from build123d import *

# Parameters (mm, degrees)
BOSS_EXTRUDE1_DEPTH      = 13
BOSS_EXTRUDE1_DEPTH_BACK = 13
SKETCH1_W                = 142.3
SKETCH1_H                = 46.5
FILLET1_R                = 1.5
SKETCH2_R                = 2.25
BOSS_EXTRUDE2_DEPTH      = 18.5
SKETCH3_R                = 0.75
BOSS_EXTRUDE3_DEPTH      = 9


with BuildPart() as part:
    # Sketch1 → Boss-Extrude1 (new, two sides: drawn at the far end of the back side and taken through both)
    with BuildSketch(Plane.XY.offset(-BOSS_EXTRUDE1_DEPTH_BACK)):
        Rectangle(SKETCH1_W, SKETCH1_H)
    extrude(amount=BOSS_EXTRUDE1_DEPTH + BOSS_EXTRUDE1_DEPTH_BACK)

    # Fillet1
    fillet1_edges = [part.edges().sort_by_distance(p)[0] for p in [
        (-71.15, 0, 13),
        (71.15, 0, -13),
        (0, -23.25, 13),
        (71.15, 0, 13),
        (0, 23.25, 13),
        (0, 23.25, -13),
        (-71.15, 0, -13),
        (-71.15, 23.25, 0),
        (71.15, 23.25, 0),
        (71.15, -23.25, 0),
        (-71.15, -23.25, 0),
        (0, -23.25, -13),
    ]]
    fillet(fillet1_edges, radius=FILLET1_R)

    # Sketch2 → Boss-Extrude2 (add)
    with BuildSketch(Plane.XY.offset(13)):
        with Locations(Location((-66.4, -18.25, 0), (0, 0, 180))):
            Circle(SKETCH2_R)
        with Locations(Location((-66.4, -13.25, 0), (0, 0, 180))):
            Circle(SKETCH2_R)
    extrude(amount=BOSS_EXTRUDE2_DEPTH)

    # Sketch3 → Boss-Extrude3 (add)
    with BuildSketch(Plane.XY.offset(13)):
        with Locations(Location((-67.9, 19.5, 0), (0, 0, 180))):
            Circle(SKETCH3_R)
        with Locations(Location((-67.9, 17.5, 0), (0, 0, 180))):
            Circle(SKETCH3_R)
        with Locations(Location((-67.9, 15.5, 0), (0, 0, 180))):
            Circle(SKETCH3_R)
    extrude(amount=BOSS_EXTRUDE3_DEPTH)


solid = part.part
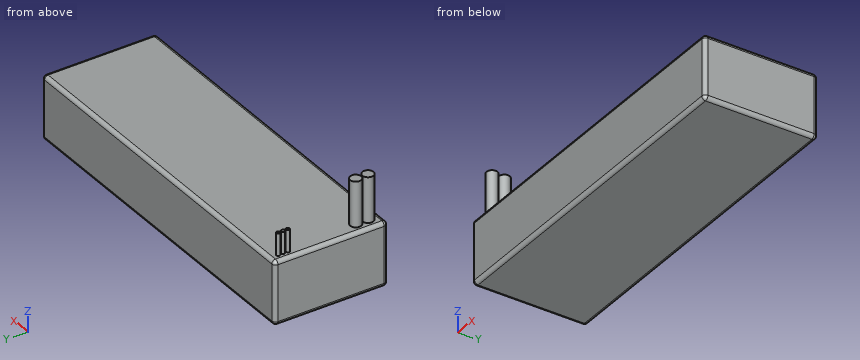
Part model, mm, in its own coordinate system. Give positions to 0.01 mm unless a question says otherwise; leave off trailing zeros. Write each loop counter-clockwise with the first axis right and the second up, starting at its lowest first coordinate (ties: lowest second). Pieces come first, ordered by that corner, then holes.
1) Cut at B-B on y = -18.25. Write the cut outline in (x, z), then the cut area to 3 significant figures.
Resolved:
outline: (-71.15, -11.5) arc R1.5 ccw to (-69.65, -13) - (69.65, -13) arc R1.5 ccw to (71.15, -11.5) - (71.15, 11.5) arc R1.5 ccw to (69.65, 13) - (-64.15, 13) - (-64.15, 31.5) - (-68.65, 31.5) - (-68.65, 13) - (-69.65, 13) arc R1.5 ccw to (-71.15, 11.5) - close
area: 3,780 mm2
2) Cut at A-A on y = -8.5. Write the cut outline in (x, z).
Resolved:
outline: (-71.15, -11.5) arc R1.5 ccw to (-69.65, -13) - (69.65, -13) arc R1.5 ccw to (71.15, -11.5) - (71.15, 11.5) arc R1.5 ccw to (69.65, 13) - (-69.65, 13) arc R1.5 ccw to (-71.15, 11.5) - close
3) Pin check, flat tips, straight feed: pin 1 (1.2 mm diameter, centred on x = -68, y = 17.5, fed in from +Z); pin 2 (10 mm diameter, centred on y = 5.5, z = 17, fed in from +X); pin 3 (8 mm diameter, centred on x = 8, y = 18.5, fed in from +Z). Stop position of each tip, or through.
Resolved:
pin 1: stops at z = 22
pin 2: stops at x = 71.06
pin 3: stops at z = 13
4) Probe L1, parallel to Z at x = 65, y = 4.5; L2, parallel to X at y = -20, z = 22. List the from-to ranges inside material, lowest first.
Resolved:
L1: z = -13 to 13
L2: x = -67.81 to -64.99
